CAD build for the part. Positions are in the model's coordinates, mm. A direction names the side the tool comes from. Give positions to 0.01 mm unless a question says otherwise; leave off trailing zeros. Loops run counter-clockwise (first coordinate to the right, second up) from the corner with the lowest first, then second, coordinate; pieces in that order, holes last. Notation, with made-up numbers: M 67.25,1.5 L 126.25,1.5 A20 cw 126.25,27.5 Z; hole C 10,22 d9. An arc over 180 degrees is marked long. Answer as CSV lines item,"result".
from build123d import *

# Parameters (mm, degrees)
SKETCH005_R  = 12
PAD004_DEPTH = 37
SKETCH006_R  = 2.75
PAD005_DEPTH = 8
SKETCH007_R  = 5.25
PAD006_DEPTH = 5


with BuildPart() as part:
    # Sketch005 → Pad004 (new body)
    with BuildSketch(Plane.YZ):
        Circle(SKETCH005_R)
    extrude(amount=PAD004_DEPTH)

    # Sketch006 (on Face3 of Pad004) → Pad005 (join)
    with BuildSketch(Plane.YZ.offset(37)):
        Circle(SKETCH006_R)
    extrude(amount=PAD005_DEPTH)

    # Sketch007 (on Face2 of Pad005) → Pad006 (join)
    with BuildSketch(Plane(origin=(0, 0, 0), x_dir=(0, 1, 0), z_dir=(-1, 0, 0))):
        Circle(SKETCH007_R)
    extrude(amount=PAD006_DEPTH)


with BuildPart() as part_1:
    # Body002 placement: moved
    add(part.part.moved(Location((12, -38, 17))))


solid = part_1.part
1) Band-saw the part on A-A on z = 17. Give the cut face in (x, y).
Answer below:
outline,"M 7,-43.25 L 12,-43.25 L 12,-50 L 49,-50 L 49,-40.75 L 57,-40.75 L 57,-35.25 L 49,-35.25 L 49,-26 L 12,-26 L 12,-32.75 L 7,-32.75 Z"
2) Which spindle directions (+Z, -Z, +X, -X, +Y, -Y) get a long thin tool onto all of the face, cutting with end or side? Do faces 1 (the face through (52.944, -40.747, 17.121)), 2 (the face through (7, -38, 17)), 3 (the face through (12, -32.8, 14.5)). Say none if no direction does.
Answer below:
face 1,"+X"
face 2,"+Z, -Z, -X, +Y, -Y"
face 3,"-X"
3) Band-saw the part on D-D on z = 20.25. Give the cut face in (x, y).
Answer below:
outline,"M 7,-42.12 L 12,-42.12 L 12,-49.55 L 49,-49.55 L 49,-26.45 L 12,-26.45 L 12,-33.88 L 7,-33.88 Z"
4) Band-saw the part on B-B on y = -38. Give the cut face in (x, z).
Answer below:
outline,"M 7,11.75 L 12,11.75 L 12,5 L 49,5 L 49,14.25 L 57,14.25 L 57,19.75 L 49,19.75 L 49,29 L 12,29 L 12,22.25 L 7,22.25 Z"
5) Flat gauge pins, fed straight in: pin 1 (1 mm diameter, centred on x = 31.5, y = -30, fed in from -Z); pin 2 (4 mm diameter, centred on y = -45.5, z = 8, fed in from -X); pin 3 (2 mm diameter, centred on x = 22, z = 22, fed in from -Y). Where does each tip first touch, or does it go through?
Answer below:
pin 1,"stops at z = 7.63"
pin 2,"stops at x = 12"
pin 3,"stops at y = -49.31"
6) Band-saw the part on C-C on x = 18. Give the cut face in (y, z), and give its area (3 significant figures).
Answer below:
outline,"C -38,17 d24"
area,"452 mm^2"
7) Drill centre lines: line 1 (X direction, y = -36.5, z = 27.75); line 2 (Z direction, x = 29, y = -38.25); line 3 (Y direction, x = 11, z = 18.5). Where is each one in solid material? Low to high. Write a range as from..to.
Answer below:
line 1,"x = 12..49"
line 2,"z = 5..29"
line 3,"y = -43.03..-32.97"
